```python
from build123d import *

# Parameters (mm, degrees)
F0_R     = 38.1
F1_DEPTH = 177.8
F1_TAPER = -7
F2_T     = -2.54
F3_W     = 139.5735256374
F3_H     = 170.4298052937
F4_DEPTH = 2.54


# Not quite as in the source:
# - a feature names something its author has since deleted; it is built from what else it names


with BuildPart() as f1:
    # F0 (on Top) → F1 (new body)
    with BuildSketch(Plane.XY):
        Circle(F0_R)
    extrude(amount=F1_DEPTH, taper=F1_TAPER)

    # F2
    f2_openings = [f1.faces().sort_by_distance(p)[0] for p in [
        (0, 0, 177.8),
    ]]
    offset(amount=F2_T, openings=f2_openings, kind=Kind.INTERSECTION)

    # F3 (on Right) → F4 (join)
    with BuildSketch(Plane.YZ):
        with Locations((10.8456704766, 92.2188116238)):
            Rectangle(F3_W, F3_H)
    extrude(amount=F4_DEPTH)


solid = f1.part
```
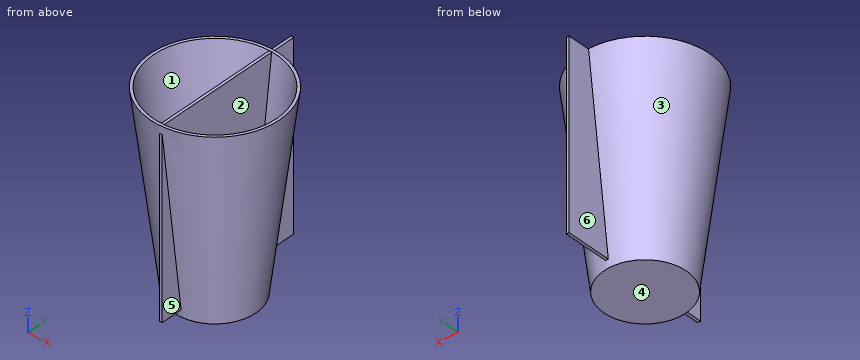
Geometry check sheet. Reference: the model listing, model coordinates, mm. Face numbers are marked on the shaded views. A direction names the side the tool comes from. Round coordinates to 2 decimals unless told otherwise and drop trailing zeros. Order: outer loops, then holes, each group sorted by start corner. A loop starts at its lowest first (then second) coordinate and runs counter-clockwise, first axis right, second up. Notation, with made-up numbers: M 19,67.5 L 59,67.5 A25 ccw 59,90.5 Z; hole C 76,41.5 d3. An arc over 180 degrees is marked long. Answer as CSV lines item,"result".
1) Tool access check on the marked faces 5 and 6. Record the directions out of +Z, -Z, +X, -X, +Y, -Y that give a thin tool (end or side, any length) a straight path to the whole face; none if there is none.
Entries:
face 5,"-Z, +X, -Y"
face 6,"-Z, -X, +Y"
2) Gauge pin test, flat ends, axial feed: pin 1 Ø0.8 at (x, y) = (1, -52.5) entering from -Z; pin 2 Ø3 at (x, y) = (1, 67.5) entering from +Z; pin 3 Ø12 at (x, z) = (-5, 75.5) entering from -Y. Record the tip position at first contact, or that the pin passes through.
Entries:
pin 1,"z = 7"
pin 2,"z = 177.43"
pin 3,"y = -58.94"
3) Mould release check, pull along X, two halves, no side actions. Record for the marked faces 1, 2, 3 and 4: +X half, -X half, draft (parallel to the pull), parting line (faces both ways), or undercut.
Entries:
face 1,"undercut"
face 2,"undercut"
face 3,"parting line"
face 4,"draft"
4) Sectioned sample at A-A on z = 160. Record the cut outline in (x, y).
Entries:
outline,"M 0,-58.94 L 2.54,-58.94 L 2.54,-57.69 A57.75 ccw 2.54,57.69 L 2.54,80.63 L 0,80.63 L 0,57.75 A57.75 ccw 0,-57.75 Z; hole M 0,-55.19 L 0,55.19 A55.19 ccw Z; hole M 2.54,-55.13 A55.19 ccw 2.54,55.13 Z"
5) Thickness scan on probe 1 along X at (y, z) = (7, 86.5); probe 2 along X at (y, z) = (-15.5, 103); probe 3 along Z at (x, y) = (11.5, -8). Record the ranges inside material, lowest first. Write a range as [from, to].
Entries:
probe 1,"[-48.22, -45.63], [0, 2.54], [45.63, 48.22]"
probe 2,"[-48.32, -45.63], [0, 2.54], [45.63, 48.32]"
probe 3,"[0, 2.54]"
6) Sectioned sample at C-C on z = 38. Record the cut outline in (x, y).
Entries:
outline,"M 0,-58.94 L 2.54,-58.94 L 2.54,-42.69 A42.77 ccw 2.54,42.69 L 2.54,80.63 L 0,80.63 L 0,42.77 A42.77 ccw 0,-42.77 Z; hole M 0,-40.21 L 0,40.21 A40.21 ccw Z; hole M 2.54,-40.13 A40.21 ccw 2.54,40.13 Z"
7) Sectioned sample at B-B on y = 67.5. Record the cut outline in (x, z), and give its area (3 significant figures).
Entries:
outline,"M 0,7 L 2.54,7 L 2.54,177.43 L 0,177.43 Z"
area,"433 mm2"
